```python
from build123d import *

# Parameters (mm, degrees)
SALIENTE_EXTRUIR1_DEPTH = 10.1
CORTAR_EXTRUIR1_DEPTH   = 10.1
REDONDEO1_R             = 2
CROQUIS3_R              = 2
CORTAR_EXTRUIR2_DEPTH   = 10.1


with BuildPart() as part:
    # Croquis1 → Saliente-Extruir1 (new body)
    with BuildSketch(Plane.XY):
        with BuildLine():
            Line((84.879626458, -20), (-27.620373542, -20))
            Line((-27.620373542, -20), (-27.620373542, 81.07249842))
            Line((-27.620373542, 81.07249842), (-27.620373542, 143))
            Line((-27.620373542, 143), (-7.620373542, 143))
            Line((-7.620373542, 143), (-7.620373542, 81.07249842))
            Line((-7.620373542, 81.07249842), (84.879626458, 0))
            Line((84.879626458, 0), (130.379626458, 0))
            ThreePointArc((130.379626458, 0), (140.379626458, -10), (130.379626458, -20))
            Line((130.379626458, -20), (84.879626458, -20))
        make_face()
    extrude(amount=SALIENTE_EXTRUIR1_DEPTH)

    # Croquis2 → Cortar-Extruir1 (cut)
    with BuildSketch(Plane.XY.offset(10.1)):
        Polygon((-7.620373542, 61.46249842), (-7.620373542, 0), (65.269626458, 0), align=None)
    extrude(amount=-CORTAR_EXTRUIR1_DEPTH, mode=Mode.SUBTRACT)

    # Redondeo1
    redondeo1_edges = [part.edges().sort_by_distance(p)[0] for p in [
        (-7.620373542, 112.03624921, 0),
        (38.629626458, 40.53624921, 0),
        (107.629626458, 0, 0),
        (140.379626458, -10, 0),
        (107.629626458, 0, 10.1),
        (38.629626458, 40.53624921, 10.1),
        (-7.620373542, 112.03624921, 10.1),
        (-27.620373542, 61.5, 10.1),
        (-7.620373542, 30.73124921, 0),
        (28.824626458, 30.73124921, 10.1),
        (28.824626458, 0, 0),
        (28.824626458, 30.73124921, 0),
        (-7.620373542, 30.73124921, 10.1),
        (28.824626458, 0, 10.1),
        (51.379626458, -20, 10.1),
        (140.379626458, -10, 10.1),
        (51.379626458, -20, 0),
        (-27.620373542, 61.5, 0),
    ]]
    fillet(redondeo1_edges, radius=REDONDEO1_R)

    # Croquis3 → Cortar-Extruir2 (cut)
    with BuildSketch(Plane.XY.offset(10.1)):
        with Locations((130.379626458, -10)):
            Circle(CROQUIS3_R)
        with Locations((-19.903008845, -12.282635303)):
            Circle(CROQUIS3_R)
        with Locations((-17.620373542, 138.637591641)):
            Circle(CROQUIS3_R)
    extrude(amount=-CORTAR_EXTRUIR2_DEPTH, mode=Mode.SUBTRACT)


solid = part.part
```
Input: part model. Units: mm. Frame: model coordinates. A direction names the side the tool comes from. Give positions to 0.01 mm unless a question says otherwise; leave off trailing zeros. Order: outer loops, then holes, each group sorted by start corner. A loop starts at its lowest first (then second) coordinate and runs counter-clockwise, first axis right, second up. Notation, with made-up numbers: (-19.5, 26) - (12.5, 26) arc R18 ccw to (12.5, 47) - close; hole circle Ø11 at (-8.75, 49.25). An arc over 180 degrees is marked (long way). Use a Markdown table: item, result.
(1) Section query A-A (x = 95.5). Output: boundary loops of the cut face in (y, z).
Computed values:
| item | result |
|---|---|
| outline | (-20, 2) arc R2 ccw to (-18, 0) - (-2, 0) arc R2 ccw to (0, 2) - (0, 8.1) arc R2 ccw to (-2, 10.1) - (-18, 10.1) arc R2 ccw to (-20, 8.1) - close |
(2) Line query: line 1 (Y direction, x = -18.5, z = 2); line 2 (Y direction, x = 108, z = 5.25); line 3 (Y direction, x = 32, z = 5). Output: solid intervals per line, ascending. Write a range as from..to.
Computed values:
| item | result |
|---|---|
| line 1 | y = -20..-13.71, -10.86..136.84, 140.43..143 |
| line 2 | y = -20..0 |
| line 3 | y = -20..0, 28.05..46.35 |
(3) Draft query along X for faces 6 (the flat face through (-18, 143, 5)), 7 (the cylindrical face through (-16.7, 136.86, 5.12)), 8 (the flat face through (-27.62, 60, 5)). Return one class per face: released by +X, released by -X, zero draft, split by the parting line, or undercut.
Computed values:
| item | result |
|---|---|
| face 6 | zero draft |
| face 7 | undercut |
| face 8 | released by -X |
(4) Pin query (flat end, axial travel): pin 1 (3 mm diameter, centred on y = 118, z = 3, fed in from +X); pin 2 (1.8 mm diameter, centred on x = 117.5, z = 6.5, fed in from +Y); pin 3 (3 mm diameter, centred on y = 26, z = 4, fed in from +X). Return the tip coordinate at first contact, or that it passes through.
Computed values:
| item | result |
|---|---|
| pin 1 | stops at x = -7.62 |
| pin 2 | stops at y = 0 |
| pin 3 | stops at x = 56.93 |
(5) Section query B-B (y = 117). Output: boundary loops of the cut face in (x, z), then the cut area to 3 significant figures.
Computed values:
| item | result |
|---|---|
| outline | (-27.62, 2) arc R2 ccw to (-25.62, 0) - (-9.62, 0) arc R2 ccw to (-7.62, 2) - (-7.62, 8.1) arc R2 ccw to (-9.62, 10.1) - (-25.62, 10.1) arc R2 ccw to (-27.62, 8.1) - close |
| area | 199 mm2 |
(6) Access query for faces 1 (the flat face through (28, 0, 5)), 2 (the cylindrical face through (29.098, 31.288, 0.57)), 3 (the cylindrical face through (140.377, -9.78, 5.007)), 4 (the cylindrical face through (29.098, 31.288, 9.53)), 5 (the flat face through (-7.62, 112, 5)). Directions: +Z, -Z, +X, -X, +Y, -Y. A direction counts if a zero-diameter tool reaches every point of the face in a straight line with its end or side. Return the directions, or none.
Computed values:
| item | result |
|---|---|
| face 1 | +Z, -Z |
| face 2 | -Z |
| face 3 | +Z, -Z, +X |
| face 4 | +Z |
| face 5 | +Z, -Z, +X, +Y |
